```python
from build123d import *

# Parameters (mm, degrees)
SALIENTE_EXTRUIR1_DEPTH      = 22.4
REDONDEO1_R                  = 1
TALADRO_DE_MARGEN_PARA_M31_D = 3.4


with BuildPart() as part:
    # Croquis1 → Saliente-Extruir1 (new, symmetric)
    with BuildSketch(Plane(origin=(0, 0, 0), x_dir=(0, 1, 0), z_dir=(0, 0, 1))):
        Polygon((-5, 13), (5, 13), (5, 5.5), (2.5, 5.5), (2.5, -5.5), (5, -5.5), (5, -13), (-5, -13), (-5, -5.5), (-2.5, -5.5), (-2.5, 5.5), (-5, 5.5), align=None)
    extrude(amount=SALIENTE_EXTRUIR1_DEPTH, both=True)

    # Redondeo1
    redondeo1_edges = [part.edges().sort_by_distance(p)[0] for p in [
        (-5.5, -5, 0),
        (-13, -5, 0),
        (-13, 5, 0),
        (-5.5, 5, 0),
        (-5.5, 2.5, 0),
        (5.5, 2.5, 0),
        (5.5, 5, 0),
        (13, 5, 0),
        (13, -5, 0),
        (5.5, -5, 0),
        (5.5, -2.5, 0),
        (-5.5, -2.5, 0),
    ]]
    fillet(redondeo1_edges, radius=REDONDEO1_R)

    # Taladro de margen para M31 (through all)
    with Locations(Plane(origin=(0, 0, -22.4), x_dir=(1, 0, 0), z_dir=(0, 0, -1))):
        with Locations((9.25, 0), (-9.25, 0)):
            Hole(TALADRO_DE_MARGEN_PARA_M31_D / 2)


solid = part.part
```
Work out the finished part from the listing and answer in its coordinate system (mm). A direction names the side the tool comes from. Round coordinates to 2 decimals unless told otherwise and drop trailing zeros. Loops run counter-clockwise (first coordinate to the right, second up) from the corner with the lowest first, then second, coordinate; pieces in that order, holes last. Notation, with made-up numbers: M 57,19 L 93,19 A22 ccw 93,46 Z; hole C 76,48 d4. An arc over 180 degrees is marked long. One line per question, with ' | ' between items.
Q1. The mould has two halves that part along X. Classify faces 4 (the flat face through (-9, -5, 0)), 5 (the cylindrical face through (5.215, 2.801, -0.314)), 6 (the cylindrical face through (-12.715, 4.699, -0.314)): +X half, -X half, draft (parallel to the pull), parting line (faces both ways), or undercut.
Conclusion:
face 4: draft | face 5: undercut | face 6: -X half
Q2. Find section D-D, the plane y = -3. Give the vertices of the cut face in (x, z), then the cut area to 3 significant figures.
Conclusion:
outline: M -13,-22.4 L -5.37,-22.4 L -5.37,22.4 L -13,22.4 Z; M 5.37,-22.4 L 13,-22.4 L 13,22.4 L 5.37,22.4 Z | area: 684 mm2
Q3. Consider line 1 along X through (y, z) = (-3.75, -18.5); line 2 along Y through (x, z) = (-9.25, 6); line 3 along Y through (x, z) = (-8.5, -11). Determine where each line is inside the solid, lowest interval first. Write a range as from..to.
Conclusion:
line 1: x = -13..-5.5, 5.5..13 | line 2: y = -5..-1.7, 1.7..5 | line 3: y = -5..-1.53, 1.53..5
Q4. A tool of negligible diameter and unlimited length cuts with its end or side. For faces 1 (the cylindrical face through (-5.785, 4.699, -0.314)), 2 (the cylindrical face through (10.6, 1.03, 0.31)), 3 (the cylindrical face through (-5.785, -4.699, 0.314)), from which of +Z, -Z, +X, -X, +Y, -Y can it reach the whole face along a straight path? Write none if from no direction.
Conclusion:
face 1: +Z, -Z, +Y | face 2: +Z, -Z | face 3: +Z, -Z, -Y
Q5. Find section A-A, the plane y = 0. Give the vertices of the cut face in (x, z).
Conclusion:
outline: M -13,-22.4 L -10.95,-22.4 L -10.95,22.4 L -13,22.4 Z; M -7.55,-22.4 L 7.55,-22.4 L 7.55,22.4 L -7.55,22.4 Z; M 10.95,-22.4 L 13,-22.4 L 13,22.4 L 10.95,22.4 Z
Q6. Each of these flat-tipped pins is pushed along its axis until it touches: pin 1 Ø5 at (x, z) = (4.5, 7) entering from -Y; pin 2 Ø7 at (x, z) = (-1, 7) entering from -Y. Where does it stop, or does it pass through?
Conclusion:
pin 1: stops at y = -5 | pin 2: stops at y = -2.5
Q7. Find section C-C, the plane z = 15. Give the vertices of the cut face in (x, y), then the cut area to 3 significant figures.
Conclusion:
outline: M -13,-4 A1 ccw -12,-5 L -6.5,-5 A1 ccw -5.5,-4 L -5.5,-3.5 A1 cw -4.5,-2.5 L 4.5,-2.5 A1 cw 5.5,-3.5 L 5.5,-4 A1 ccw 6.5,-5 L 12,-5 A1 ccw 13,-4 L 13,4 A1 ccw 12,5 L 6.5,5 A1 ccw 5.5,4 L 5.5,3.5 A1 cw 4.5,2.5 L -4.5,2.5 A1 cw -5.5,3.5 L -5.5,4 A1 ccw -6.5,5 L -12,5 A1 ccw -13,4 Z; hole C -9.25,0 d3.4; hole C 9.25,0 d3.4 | area: 186 mm2
Q8. Find section B-B, the plane x = 9.25. Give the vertices of the cut face in (y, z).
Conclusion:
outline: M -5,-22.4 L -1.7,-22.4 L -1.7,22.4 L -5,22.4 Z; M 1.7,-22.4 L 5,-22.4 L 5,22.4 L 1.7,22.4 Z
